```python
from build123d import *

# Parameters (mm, degrees)
BOSS_EXTRUDE1_DEPTH = 76.2
SKETCH2_R           = 44.45
BOSS_EXTRUDE2_DEPTH = 3.175


with BuildPart() as part:
    # Sketch1 → Boss-Extrude1 (new body)
    with BuildSketch(Plane.XY):
        Polygon((7.332348419, 0), (3.666174209, 6.35), (-3.666174209, 6.35), (-7.332348419, 0), (-3.666174209, -6.35), (3.666174209, -6.35), align=None)
    extrude(amount=-BOSS_EXTRUDE1_DEPTH)

    # Sketch2 → Boss-Extrude2 (add)
    with BuildSketch(Plane.XY):
        Circle(SKETCH2_R)
    extrude(amount=BOSS_EXTRUDE2_DEPTH)


solid = part.part
```
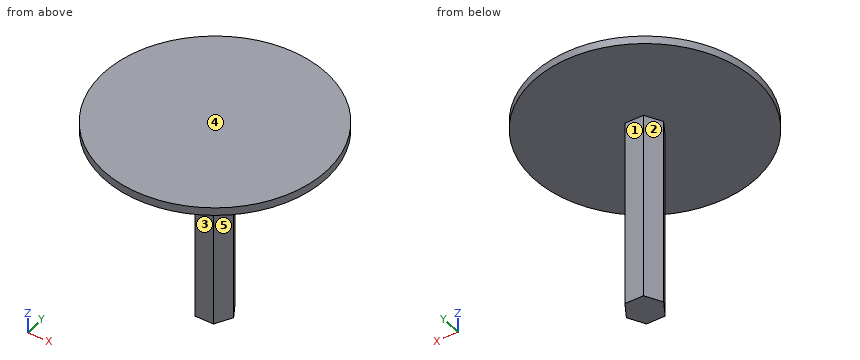
Design review of the part built by this model. Coordinates are the model's own, in mm. Face numbers are marked on the shaded views. A direction names the side the tool comes from. Round coordinates to 2 decimals unless told otherwise and drop trailing zeros. Write each loop counter-clockwise with the first axis right and the second up, starting at its lowest first coordinate (ties: lowest second). Pieces come first, ordered by that corner, then holes.
Item 1: For probe 1 along Z at (x, y) = (-39, -6) (3 decimals); probe 2 along X at (y, z) = (-5, -40); probe 3 along Y at (x, z) = (-0.5, -1), list the stretches that pass through material, from the lowest coordinate up.
Item 2: For the marked faces 1, 2, 3, 4 and 5, list the 3-axis set-ups (+Z, -Z, +X, -X, +Y, -Y) from which the entire face can be reached by the end or side of a thin tool; tool diameter is ignored.
Item 3: We need section A-A on z = -70. Write out the cut boundary in (x, y), and give its area (3 significant figures).
Item 4: Clearance check with flat-ended pins moving along their axes: pin 1 Ø2 at (x, z) = (1, -20.5) entering from -Y; pin 2 Ø4 at (y, z) = (8, -33.5) entering from -X; pin 3 Ø3.5 at (x, z) = (-1.5, -23) entering from +Y. State where each tip first meets the part, or that it passes through.
Item 5: We need section C-C on y = -34. Write out the cut boundary in (x, z) (3 decimals), and give its area (3 significant figures).
Item 6: We need section B-B on x = 0. Write out the cut boundary in (y, z) (3 decimals).
Item 7: We need section D-D on y = 29.5. Write out the cut boundary in (x, z) (3 decimals).
Returned:
1. probe 1: z = 0 to 3.175
1. probe 2: x = -4.45 to 4.45
1. probe 3: y = -6.35 to 6.35
2. face 1: -Z, +X, -X, +Y
2. face 2: -Z, -X, +Y
2. face 3: -Z, +X, -X, -Y
2. face 4: +Z, +X, -X, +Y, -Y
2. face 5: -Z, +X, -Y
3. outline: (-7.33, 0) - (-3.67, -6.35) - (3.67, -6.35) - (7.33, 0) - (3.67, 6.35) - (-3.67, 6.35) - close
3. area: 140 mm2
4. pin 1: stops at y = -6.35
4. pin 2: stops at x = -3.87
4. pin 3: stops at y = 6.35
5. outline: (-28.632, 0) - (28.632, 0) - (28.632, 3.175) - (-28.632, 3.175) - close
5. area: 182 mm2
6. outline: (-44.45, 0) - (-6.35, 0) - (-6.35, -76.2) - (6.35, -76.2) - (6.35, 0) - (44.45, 0) - (44.45, 3.175) - (-44.45, 3.175) - close
7. outline: (-33.25, 0) - (33.25, 0) - (33.25, 3.175) - (-33.25, 3.175) - close
